Could you check a few things on this model? Use its own coordinates, in mm. A direction names the side the tool comes from. Coordinates: 2 decimals unless noted, no trailing zeros. Write each loop counter-clockwise with the first axis right and the second up, starting at its lowest first coordinate (ties: lowest second). Pieces come first, ordered by that corner, then holes.
Item 1: Which directions (+Z, -Z, +X, -X, +Y, -Y) give clear straight access to the entire face, cutting with the end or side of a thin tool? Please do faces 4 (the flat face through (-28.774, 49.415, -3.585)), 5 (the cylindrical face through (-19.1, 18.4, 3.9)), 6 (the flat face through (-21.773, 49.415, -3.575)).
Item 2: I want a section at A-A on y = 36.5. Please give me the cut outline in (x, z), then the cut area to 3 significant figures.
Item 3: If I drill on probe 1 along Z at (x, y) = (-22.5, 20); probe 2 along Y at (x, z) = (-25, 11.75); probe 3 along X at (y, z) = (52.5, 6.5), over which ranges is the centre line in solid material (lowest first)?
Item 4: For P1, Ø8, axis at x = -19.5, y = 26, coming from the -Z side; P2, Ø3, axis at x = -29, y = 28.5, coming from the +Z side; P3, Ø7, axis at x = -25.5, z = 2.5, coming from the -Y side, each with a flat end and sliding along its axis, tell me the tip position at first contact or that it passes through.
Item 5: Thinking about a two-plate mould opening in X: for faces 1 (the flat face through (-23, 22.3, -4)), 2 (the flat face through (-19.93, 3.5, 2)), 3 (the flat face through (-30.17, 3.5, -4.47)), which applies, +X half, -X half, draft (parallel to the pull), parting line (faces both ways), or undercut?
Item 6: I want a section at B-B on y = 18.5. Please give me the cut outline in (x, z), then the cut area to 3 significant figures.
from build123d import *

# Parameters (mm, degrees)
BOSS_EXTRUDE1_DEPTH = 7.1
SKETCH2_R           = 7.682494309
SKETCH2_R_2         = 1.75
BOSS_EXTRUDE3_DEPTH = 7.6
BOSS_EXTRUDE3_DRAFT = 10
SKETCH6_R           = 6.342409255
BOSS_EXTRUDE6_DEPTH = 7.6
BOSS_EXTRUDE7_DEPTH = 55


with BuildPart() as part:
    # Sketch1 → Boss-Extrude1 (new body)
    with BuildSketch(Plane(origin=(0, 0, 0), x_dir=(1, 0, 0), z_dir=(0, 1, 0))):
        Polygon((-17.299814282, 3.228425178), (-26.236838815, 7.285878299), (-34.219208559, 1.57491458), (-33.26455377, -8.193502261), (-24.327529237, -12.250955382), (-16.345159493, -6.539991662), align=None)
        Polygon((-19.630317243, -5.048513876), (-20.234050809, 1.129134004), (-25.885917592, 3.695109339), (-30.934050809, 0.083436793), (-30.330317243, -6.094211087), (-24.67845046, -8.660186422), align=None, mode=Mode.SUBTRACT)
    extrude(amount=BOSS_EXTRUDE1_DEPTH)


with BuildPart() as boss_extrude3_tool:
    # Sketch2 → Boss-Extrude3 (with draft: the straight prism first)
    with BuildSketch(Plane(origin=(0, 7.1, 0), x_dir=(1, 0, 0), z_dir=(0, 1, 0))):
        with Locations((-25.282184026, -2.482538541)):
            Circle(SKETCH2_R)
        with Locations((-25.282184026, -2.482538541)):
            Circle(SKETCH2_R_2, mode=Mode.SUBTRACT)
    extrude(amount=BOSS_EXTRUDE3_DEPTH)
    # Boss-Extrude3: the draft: its side faces are tilted about the plane it starts from
    boss_extrude3_sides = [boss_extrude3_tool.faces().sort_by_distance(p)[0] for p in [
        (-32.964678335, 10.9, 2.482538541),
        (-27.032184026, 10.9, 2.482538541),
    ]]
    draft(boss_extrude3_sides, Plane(origin=(0, 7.1, 0), x_dir=(1, 0, 0), z_dir=(0, 1, 0)), BOSS_EXTRUDE3_DRAFT)


with BuildPart() as part_1:
    add(part.part)

    # Boss-Extrude3: add boss_extrude3_tool
    add(boss_extrude3_tool.part)

    # Sketch6 → Boss-Extrude6 (add)
    with BuildSketch(Plane(origin=(0, 14.7, 0), x_dir=(1, 0, 0), z_dir=(0, 1, 0))):
        with Locations(Location((-25.282184026, -2.482538541, 0), (0, 0, 90))):
            Circle(SKETCH6_R)
    extrude(amount=BOSS_EXTRUDE6_DEPTH)

    # Sketch7 → Boss-Extrude7 (add)
    with BuildSketch(Plane(origin=(0, 22.3, 0), x_dir=(1, 0, 0), z_dir=(0, 1, 0))):
        Polygon((-18.255240013, -6.477322026), (-18.309128039, 1.605581742), (-25.336072052, 5.600365227), (-32.309128039, 1.512244944), (-32.255240013, -6.570658825), (-25.228296, -10.56544231), align=None)
    extrude(amount=BOSS_EXTRUDE7_DEPTH)


solid = part_1.part
Response values:
1. face 4: -Z, -X, +Y
1. face 5: none
1. face 6: -Z, +X, +Y
2. outline: (-32.31, -1.51) - (-25.34, -5.6) - (-18.31, -1.61) - (-18.26, 6.48) - (-25.23, 10.57) - (-32.26, 6.57) - close
2. area: 170 mm2
3. probe 1: z = -3.22 to 8.18
3. probe 2: y = 0 to 7.1
3. probe 3: x = -32.26 to -18.29
4. P1: stops at z = -4.56
4. P2: stops at z = 9.27
4. P3: stops at y = 7.1
5. face 1: draft
5. face 2: undercut
5. face 3: -X half
6. outline: circle Ø12.68 at (-25.28, 2.48)
6. area: 126 mm2
